Input: part model. Units: mm. Frame: model coordinates. A direction names the side the tool comes from. Coordinates: 2 decimals unless noted, no trailing zeros. Loops run counter-clockwise (first coordinate to the right, second up) from the corner with the lowest first, then second, coordinate; pieces in that order, holes last.
```python
from build123d import *

# Parameters (mm, degrees)
SKETCH1_R             = 25.4
BOSS_EXTRUDE1_DEPTH   = 25.4
BOSS_EXTRUDE1_2_DEPTH = 25.4
SKETCH3_W             = 40.64380449
SKETCH3_H             = 30.474926688
BOSS_EXTRUDE2_DEPTH   = 152.4
SKETCH4_W             = 40.492338346
SKETCH4_H             = 30.67589502
BOSS_EXTRUDE3_DEPTH   = 152.4
SKETCH5_W             = 650.092338346
SKETCH5_H             = 304.8
SKETCH5_W_2           = 137.16
SKETCH5_H_2           = 279.4
SKETCH5_W_3           = 324.972338346
SKETCH5_H_3           = 25.4
SKETCH5_H_4           = 203.2
BOSS_EXTRUDE4_DEPTH   = 12.7


with BuildPart() as part:
    # Sketch1 → Boss-Extrude1 (new body)
    with BuildSketch(Plane(origin=(0, 0, 0), x_dir=(1, 0, 0), z_dir=(0, 1, 0))):
        with Locations(Location((304.8, 0, 0), (0, 0, 270))):
            Circle(SKETCH1_R)
    extrude(amount=BOSS_EXTRUDE1_DEPTH)

    # Sketch3 → Boss-Extrude2 (add)
    with BuildSketch(Plane(origin=(0, 25.4, 0), x_dir=(1, 0, 0), z_dir=(0, 1, 0))):
        with Locations((304.8, 0)):
            Rectangle(SKETCH3_W, SKETCH3_H)
    extrude(amount=BOSS_EXTRUDE2_DEPTH)



with BuildPart() as body_2:
    # Sketch1 → Boss-Extrude1 2 (new body)
    with BuildSketch(Plane(origin=(0, 0, 0), x_dir=(1, 0, 0), z_dir=(0, 1, 0))):
        with Locations(Location((-304.8, 0, 0), (0, 0, 270))):
            Circle(SKETCH1_R)
    extrude(amount=BOSS_EXTRUDE1_2_DEPTH)

    # Sketch4 → Boss-Extrude3 (add)
    with BuildSketch(Plane(origin=(0, 25.4, 0), x_dir=(1, 0, 0), z_dir=(0, 1, 0))):
        with Locations((-304.8, 0)):
            Rectangle(SKETCH4_W, SKETCH4_H)
    extrude(amount=BOSS_EXTRUDE3_DEPTH)


with BuildPart() as part_1:
    add(part.part)

    add(body_2.part)  # Boss-Extrude4 merges body 2
    # Sketch5 → Boss-Extrude4 (add)
    with BuildSketch(Plane(origin=(0, 177.8, 0), x_dir=(1, 0, 0), z_dir=(0, 1, 0))):
        Rectangle(SKETCH5_W, SKETCH5_H)
        with Locations((-243.766169173, 0)):
            Rectangle(SKETCH5_W_2, SKETCH5_H_2, mode=Mode.SUBTRACT)
        with Locations((243.766169173, 0)):
            Rectangle(SKETCH5_W_2, SKETCH5_H_2, mode=Mode.SUBTRACT)
        with Locations((0, 127)):
            Rectangle(SKETCH5_W_3, SKETCH5_H_3, mode=Mode.SUBTRACT)
        Rectangle(SKETCH5_W_3, SKETCH5_H_4, mode=Mode.SUBTRACT)
        with Locations((0, -127)):
            Rectangle(SKETCH5_W_3, SKETCH5_H_3, mode=Mode.SUBTRACT)
    extrude(amount=BOSS_EXTRUDE4_DEPTH)


solid = part_1.part
```
Item 1: Line query: L1, parallel to X at y = 104.5, z = 5; L2, parallel to Y at x = 7.5, z = -105; L3, parallel to Z at x = -297.5, y = 76. Output: solid intervals per line, ascending.
Result:
L1: x = -325.05 to -284.55, 284.48 to 325.12
L2: y = 177.8 to 190.5
L3: z = -15.34 to 15.34
Item 2: Reachability of faces 4 (the face through (284.478, 101, 0)), 5 (the face through (280.004, 12.522, -5.506)), 6 (the face through (-162.486, 184, 127)), 7 (the face through (-299, 177.8, 0)) from +Z, -Z, +X, -X, +Y, -Y: full face, straight path, thin tool, end or side. Return the list, or none.
Result:
face 4: +Z, -Z, +Y
face 5: -Y
face 6: +Y, -Y
face 7: +Y
Item 3: Section query B-B (x = -304.8). Output: boundary loops of the cut face in (y, z), then the cut area to 3 significant figures.
Result:
outline: (0, -25.4) - (25.4, -25.4) - (25.4, -15.34) - (177.8, -15.34) - (177.8, 15.34) - (25.4, 15.34) - (25.4, 25.4) - (0, 25.4) - close; (177.8, -152.4) - (190.5, -152.4) - (190.5, -139.7) - (177.8, -139.7) - close; (177.8, 139.7) - (190.5, 139.7) - (190.5, 152.4) - (177.8, 152.4) - close
area: 6,290 mm2
Item 4: Section query C-C (z = 0). Count the separate pieces of the cut face and the enclosed holes in it, then the cut area to 3 significant figures.
Result:
separate pieces: 4
enclosed holes: 0
area: 15,600 mm2
Item 5: Mould query, pull axis X, two halves, no side actions, for faces 1 (the face through (-245, 184, -139.7)), 2 (the face through (305, 101, 15.237)), 3 (the face through (-325.046, 132, 1)). Classes: +X half, -X half, draft (parallel to the pull), parting line (faces both ways), or undercut.
Result:
face 1: undercut
face 2: draft
face 3: -X half
Item 6: Contact query for flat-ended pins moving along their axis: P1, Ø22, axis at x = -293, z = 7.5, coming from the +Y side; P2, Ø10, axis at y = 185, z = 19, coming from the +X side; P3, Ø4, axis at y = 182.5, z = -16.5, coming from the -X side; P4, Ø8, axis at y = 171, z = 88.5, coming from the +X side. Output: stop coordinate, or through.
Result:
P1: stops at y = 177.8
P2: stops at x = 325.05
P3: stops at x = -325.05
P4: passes through
Item 7: Section query D-D (x = 29). Output: boundary loops of the cut face in (y, z), then the cut area to 3 significant figures.
Result:
outline: (177.8, -152.4) - (190.5, -152.4) - (190.5, -139.7) - (177.8, -139.7) - close; (177.8, -114.3) - (190.5, -114.3) - (190.5, -101.6) - (177.8, -101.6) - close; (177.8, 101.6) - (190.5, 101.6) - (190.5, 114.3) - (177.8, 114.3) - close; (177.8, 139.7) - (190.5, 139.7) - (190.5, 152.4) - (177.8, 152.4) - close
area: 645 mm2
Item 8: Section query A-A (y = 76). Output: boundary loops of the cut face in (x, z).
Result:
outline: (-325.05, -15.34) - (-284.55, -15.34) - (-284.55, 15.34) - (-325.05, 15.34) - close; (284.48, -15.24) - (325.12, -15.24) - (325.12, 15.24) - (284.48, 15.24) - close
